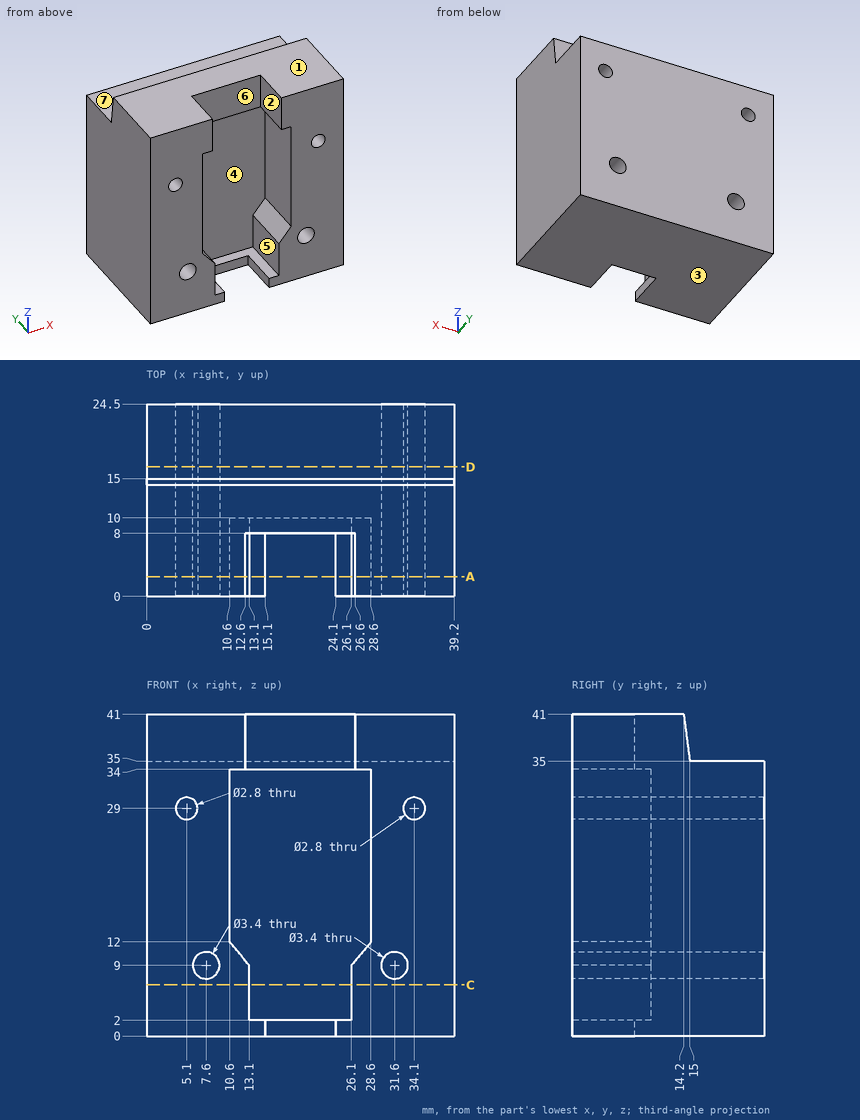
The figure shows three views and two pictorial views of one solid part (mm, origin at its lowest corner). Answer the questions. A direction names the side the tool comes from. Give positions to 0.01 mm unless a question says otherwise; leave off trailing zeros. Write each loop counter-clockwise with the first axis right and the second up, starting at its lowest first coordinate (ties: lowest second). Pieces come first, ordered by that corner, then holes. Notation, with made-up numbers: (76, -38) - (129, -38) arc R33 ccw to (129, -5) - close; hole circle Ø6 at (17, -1.75). An arc over 180 degrees is marked (long way). Return JSON: item names as keys, results as strings.
Q1. Given P1, Ø6, axis at x = 23.5, y = 19.5, coming from the +Z side; P2, Ø8, axis at x = 21, y = 3, coming from the +Z side; P3, Ø9, axis at x = 17.5, z = 21.5, coming from the -Y side, each flat-ended and moving along its own axis, determine where each tip first touches the part or whether it passes through.
Reply:
{"P1": "z = 35", "P2": "z = 2", "P3": "y = 10"}
Q2. For the marked faces 5, 6 and 7, determine the directions among +Z, -Z, +X, -X, +Y, -Y from which every point of the face is accessible in a straight line to the end or side of a thin tool.
Reply:
{"face 5": "-Y", "face 6": "+Z, -Y", "face 7": "+Z, +X, -X, +Y"}
Q3. A cutting plane is placed at D-D, the plane y = 16.5. Determine the outline of the cut face in (x, z).
Reply:
{"outline": "(0, 0) - (39.2, 0) - (39.2, 35) - (0, 35) - close; hole circle Ø2.8 at (5.1, 29); hole circle Ø3.4 at (7.6, 9); hole circle Ø3.4 at (31.6, 9); hole circle Ø2.8 at (34.1, 29)"}
Q4. A cutting plane is placed at A-A, the plane y = 2.5. Determine the outline of the cut face in (x, z), and give its area (3 significant figures).
Reply:
{"outline": "(0, 0) - (15.1, 0) - (15.1, 2) - (13.1, 2) - (13.1, 9) - (10.6, 12) - (10.6, 34) - (12.6, 34) - (12.6, 41) - (0, 41) - close; (24.1, 0) - (39.2, 0) - (39.2, 41) - (26.6, 41) - (26.6, 34) - (28.6, 34) - (28.6, 12) - (26.1, 9) - (26.1, 2) - (24.1, 2) - close; hole circle Ø2.8 at (5.1, 29); hole circle Ø3.4 at (7.6, 9); hole circle Ø3.4 at (31.6, 9); hole circle Ø2.8 at (34.1, 29)", "area": "927 mm²"}
Q5. A cutting plane is placed at C-C, the plane z = 6.5. Determine the outline of the cut face in (x, y).
Reply:
{"outline": "(0, 0) - (13.1, 0) - (13.1, 10) - (26.1, 10) - (26.1, 0) - (39.2, 0) - (39.2, 24.5) - (0, 24.5) - close"}
Q6. For a pull along Z with two mould halves and no side action, classify the marked faces 1, 2, 3 and 4 as released by +Z, released by -Z, zero draft, split by the parting line, or undercut.
Reply:
{"face 1": "released by +Z", "face 2": "zero draft", "face 3": "released by -Z", "face 4": "undercut"}
Q7. Consider line 1 along X through (y, z) = (5.75, 28); line 2 along Z through (x, y) = (7.6, 10.5); line 3 along X through (y, z) = (3.5, 12). Determine where each line is inside the solid, lowest interval first. Write a range as [from, to].
Reply:
{"line 1": "[0, 4.12], [6.08, 10.6], [28.6, 33.12], [35.08, 39.2]", "line 2": "[0, 7.3], [10.7, 41]", "line 3": "[0, 10.6], [28.6, 39.2]"}
